from build123d import *

# Parameters (mm, degrees)
ESQUISSE1_R        = 1.25
ESQUISSE1_W        = 3
ESQUISSE1_H        = 7.3
BOSS_EXTRU_1_DEPTH = 3


with BuildPart() as part:
    # Esquisse1 → Boss.-Extru.1 (new body)
    with BuildSketch(Plane(origin=(0, 0, 0), x_dir=(1, 0, 0), z_dir=(0, 1, 0))):
        with BuildLine():
            Line((-18.5, 24), (18.5, 24))
            ThreePointArc((18.5, 24), (20.621320344, 23.121320344), (21.5, 21))
            Line((21.5, 21), (21.5, 0))
            Line((21.5, 0), (-21.5, 0))
            Line((-21.5, 0), (-21.5, 21))
            ThreePointArc((-21.5, 21), (-20.621320344, 23.121320344), (-18.5, 24))
        make_face()
        with Locations(Location((-15, 20, 0), (0, 0, 270))):
            Circle(ESQUISSE1_R, mode=Mode.SUBTRACT)
        with Locations(Location((15, 20, 0), (0, 0, 270))):
            Circle(ESQUISSE1_R, mode=Mode.SUBTRACT)
        with Locations(Location((15, 4, 0), (0, 0, 270))):
            Circle(ESQUISSE1_R, mode=Mode.SUBTRACT)
        with Locations(Location((-15, 4, 0), (0, 0, 270))):
            Circle(ESQUISSE1_R, mode=Mode.SUBTRACT)
        with Locations((-10, 7.9)):
            Rectangle(ESQUISSE1_W, ESQUISSE1_H, mode=Mode.SUBTRACT)
        with Locations((10, 7.9)):
            Rectangle(ESQUISSE1_W, ESQUISSE1_H, mode=Mode.SUBTRACT)
    extrude(amount=BOSS_EXTRU_1_DEPTH)


solid = part.part
Here's how the part is built. I have some questions about the finished solid (model axes, mm). A direction names the side the tool comes from. Round coordinates to 2 decimals unless told otherwise and drop trailing zeros. Order: outer loops, then holes, each group sorted by start corner. A loop starts at its lowest first (then second) coordinate and runs counter-clockwise, first axis right, second up. Notation, with made-up numbers: M -1,48.25 L 29,48.25 A20 ccw 29,84.25 Z; hole C 64.25,-3.75 d9. An arc over 180 degrees is marked long. Return JSON: item names as keys, results as strings. Group by question number.
1. If we section it at C-C on y = 1.1: List the corners of the cut face in (x, z) for me.
2. If we section it at B-B on x = -15: List the corners of the cut face in (y, z) for me, then the cut area to 3 significant figures.
3. If we section it at A-A on z = -20: List the corners of the cut face in (x, y) for me.
4. If we mould it in two halves opening along Z, with no side actions, what happens to faces 1 (the face through (20.6, 1.48, -23.14)), 2 (the face through (-21.5, 1, -10)), 3 (the face through (-11.5, 1, -8))? For each: pulls with the +Z half, pulls with the -Z half, needs draft (parallel to the pull), parting line crosses it, or undercut.
5. On a 3-axis mill with a long thin cutter (end or side, diameter ignored), from which of +Z, -Z, +X, -X, +Y, -Y can I reach the whole of each face in a straight line? I mean faces 4 (the face through (0, 3, -12)), 5 (the face through (-8.5, 1, -8)). Say none if no direction works.
6. Please list where these lines run through material, in increasing order: probe 1 along X at (y, z) = (2.05, -4); probe 2 along X at (y, z) = (0.5, -7.25); probe 3 along X at (y, z) = (1.45, -5).
Reply:
{
 "1": {"outline": "M -21.5,-21 A3 ccw -18.5,-24 L 18.5,-24 A3 ccw 21.5,-21 L 21.5,0 L -21.5,0 Z; hole C -15,-20 d2.5; hole C -15,-4 d2.5; hole M -11.5,-11.55 L -8.5,-11.55 L -8.5,-4.25 L -11.5,-4.25 Z; hole M 8.5,-11.55 L 11.5,-11.55 L 11.5,-4.25 L 8.5,-4.25 Z; hole C 15,-20 d2.5; hole C 15,-4 d2.5"},
 "2": {"outline": "M 0,-24 L 3,-24 L 3,-21.25 L 0,-21.25 Z; M 0,-18.75 L 3,-18.75 L 3,-5.25 L 0,-5.25 Z; M 0,-2.75 L 3,-2.75 L 3,0 L 0,0 Z", "area": "57.0 mm^2"},
 "3": {"outline": "M -21.5,0 L -16.25,0 L -16.25,3 L -21.5,3 Z; M -13.75,0 L 13.75,0 L 13.75,3 L -13.75,3 Z; M 16.25,0 L 21.5,0 L 21.5,3 L 16.25,3 Z"},
 "4": {"face 1": "pulls with the -Z half", "face 2": "needs draft", "face 3": "undercut"},
 "5": {"face 4": "+Z, -Z, +X, -X, +Y", "face 5": "+Y, -Y"},
 "6": {"probe 1": "-21.5 to -16.25, -13.75 to 13.75, 16.25 to 21.5", "probe 2": "-21.5 to -11.5, -8.5 to 8.5, 11.5 to 21.5", "probe 3": "-21.5 to -15.75, -14.25 to -11.5, -8.5 to 8.5, 11.5 to 14.25, 15.75 to 21.5"}
}
